Could you check a few things on this model? Use its own coordinates, in mm. Give positions to 0.01 mm unless a question says otherwise; leave off trailing zeros. Order: outer loops, then holes, each group sorted by start corner. A loop starts at its lowest first (then second) coordinate and runs counter-clockwise, first axis right, second up. Notation, with made-up numbers: M 61,34.25 L 86,34.25 A22 cw 86,54.25 Z; hole C -27,12 d6. An arc over 180 degrees is marked long. Use a Markdown table: item, result. Add a question column.
Item 1: Suppose I cut it at B-B on z = 0. Write out the boundary of the cut face in (x, y), plus the area to 4 significant figures.
Item 2: Suppose I cut it at C-C on y = -0.3. Count the separate pieces of the cut face and the enclosed holes in it, plus the area to 3 significant figures.
Item 3: Suppose I cut it at A-A on x = 0. Write out the boundary of the cut face in (y, z).
Item 4: If we mould it in two halves opening along X, with no side actions, what happens to faces 1 (the face through (-1.147, -0.74, 28.477)), 2 (the face through (-26, 0, -48)), 3 (the face through (53.5, -0.76, -145.07))? For each: released by +X, released by -X, zero draft, split by the parting line, or undercut.
Item 5: If I drill on L1, parallel to X at y = -0.9, z = -125.5; L2, parallel to Z at x = 44.5, y = -0.45; L3, parallel to X at y = -1.05, z = 21, over which ranges is the centre line in solid material (lowest first)? Write a range as from..to.
from build123d import *

# Parameters (mm, degrees)
F0_W     = 160
F0_H     = 195
F0_R     = 1.75
F1_DEPTH = 1.5
F2_R     = 2
F3_R     = 4
F4_R     = 5


with BuildPart() as f1:
    # F0 (on Front) → F1 (new body)
    with BuildSketch(Plane.XZ):
        with Locations((-25, -49)):
            Rectangle(F0_W, F0_H)
        with Locations((-94.5, -125.5)):
            Circle(F0_R, mode=Mode.SUBTRACT)
        with Locations((-94.5, -51)):
            Circle(F0_R, mode=Mode.SUBTRACT)
        with Locations((44.5, -125.5)):
            Circle(F0_R, mode=Mode.SUBTRACT)
        with Locations((44.5, -51)):
            Circle(F0_R, mode=Mode.SUBTRACT)
        with Locations((-94.5, 23.5)):
            Circle(F0_R, mode=Mode.SUBTRACT)
        with Locations((-23.546656, -23.546656)):
            Circle(F0_R, mode=Mode.SUBTRACT)
        with BuildLine():
            ThreePointArc((-7.5, -27.495454), (0, 28.5), (7.5, -27.495454))
            Line((7.5, -27.495454), (7.5, -30))
            Line((7.5, -30), (7.5, -36.495454))
            Line((7.5, -36.495454), (3.75, -37.75))
            Line((3.75, -37.75), (0, -37.75))
            Line((0, -37.75), (-3.75, -37.75))
            Line((-3.75, -37.75), (-7.5, -36.495454))
            Line((-7.5, -36.495454), (-7.5, -30))
            Line((-7.5, -30), (-7.5, -27.495454))
        make_face(mode=Mode.SUBTRACT)
        with Locations((23.546656, -23.546656)):
            Circle(F0_R, mode=Mode.SUBTRACT)
        with Locations((-23.546656, 23.546656)):
            Circle(F0_R, mode=Mode.SUBTRACT)
        with Locations((23.546656, 23.546656)):
            Circle(F0_R, mode=Mode.SUBTRACT)
        with Locations((44.5, 23.5)):
            Circle(F0_R, mode=Mode.SUBTRACT)
    extrude(amount=F1_DEPTH)

    # F2
    f2_edges = [f1.edges().sort_by_distance(p)[0] for p in [
        (7.5, -0.75, -36.495454),
        (-7.5, -0.75, -36.495454),
    ]]
    fillet(f2_edges, radius=F2_R)

    # F3
    f3_edges = [f1.edges().sort_by_distance(p)[0] for p in [
        (3.75, -0.75, -37.75),
        (-3.75, -0.75, -37.75),
    ]]
    fillet(f3_edges, radius=F3_R)

    # F4
    f4_edges = [f1.edges().sort_by_distance(p)[0] for p in [
        (55, -0.75, 48.5),
        (-105, -0.75, 48.5),
        (-105, -0.75, -146.5),
        (55, -0.75, -146.5),
    ]]
    fillet(f4_edges, radius=F4_R)


solid = f1.part
Findings below:
| question | item | result |
|---|---|---|
| 1 | outline | M -105,-1.5 L -28.5,-1.5 L -28.5,0 L -105,0 Z; M 28.5,-1.5 L 55,-1.5 L 55,0 L 28.5,0 Z |
| 1 | area | 154.5 mm^2 |
| 2 | separate pieces | 1 |
| 2 | enclosed holes | 11 |
| 2 | area | 28,400 mm^2 |
| 3 | outline | M -1.5,-146.5 L 0,-146.5 L 0,-37.75 L -1.5,-37.75 Z; M -1.5,28.5 L 0,28.5 L 0,48.5 L -1.5,48.5 Z |
| 4 | face 1 | undercut |
| 4 | face 2 | zero draft |
| 4 | face 3 | released by +X |
| 5 | L1 | x = -105..-96.25, -92.75..42.75, 46.25..55 |
| 5 | L2 | z = -146.5..-127.25, -123.75..-52.75, -49.25..21.75, 25.25..48.5 |
| 5 | L3 | x = -105..-19.27, 19.27..55 |
